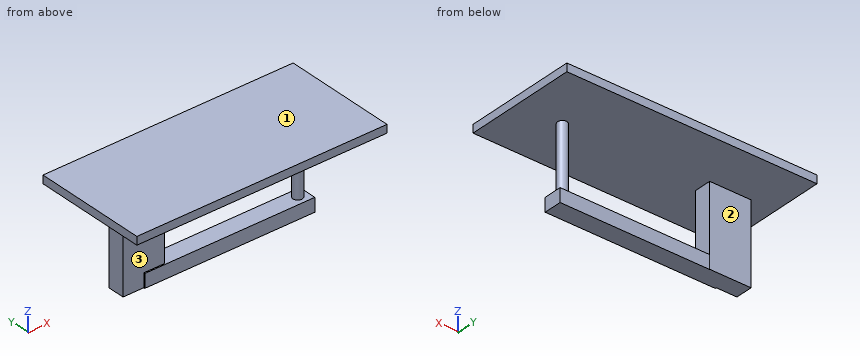
from build123d import *

# Parameters (mm, degrees)
F0_W     = 89.621424675
F0_H     = 36.9273871183
F1_DEPTH = 174.3299812078
F3_W     = 541.3100868464
F3_H     = 245.468556881
F4_DEPTH = 17.3550322652
F2_W     = 38.959980011
F2_H     = 29.5604169369
F5_DEPTH = 368.040561676
F6_R     = 10.2494359016
F7_DEPTH = 180.2812367678


with BuildPart() as f1:
    # F0 (on Top) → F1 (new body)
    with BuildSketch(Plane.XY):
        with Locations((0, 18.4636935592)):
            Rectangle(F0_W, F0_H)
    extrude(amount=F1_DEPTH)

    # F3 (on face) → F4 (join)
    with BuildSketch(Plane.XY.offset(174.3299812078)):
        with Locations((172.7937683463, 22.5193798542)):
            Rectangle(F3_W, F3_H)
    extrude(amount=F4_DEPTH)

    # F2 (on Right) → F5 (join)
    with BuildSketch(Plane.YZ):
        with Locations((16.8825984001, 14.7802084684)):
            Rectangle(F2_W, F2_H)
    extrude(amount=F5_DEPTH)

    # F6 (on face) → F7 (join)
    with BuildSketch(Plane(origin=(0, 0, 0), x_dir=(1, 0, 0), z_dir=(0, 0, -1))):
        with Locations((347.0340669155, -16.8822109699)):
            Circle(F6_R)
    extrude(amount=-F7_DEPTH)


solid = f1.part
The listing builds one solid part. Answer for the finished solid, in the listing's coordinates (mm). Face numbers are marked on the shaded views. Coordinates: 2 decimals unless noted, no trailing zeros. Write each loop counter-clockwise with the first axis right and the second up, starting at its lowest first coordinate (ties: lowest second). Pieces come first, ordered by that corner, then holes. Notation, with made-up numbers: (-32.75, 55) - (-22.75, 55) arc R13 cw to (-22.75, 72) - close; hole circle Ø9 at (52.5, 22). An arc over 180 degrees is marked (long way). Return JSON: item names as keys, results as strings.
1. The part is cut by section D-D on z = 141.5. Determine the outline of the cut face in (x, y).
Final values:
{"outline": "(-44.81, 0) - (44.81, 0) - (44.81, 36.93) - (-44.81, 36.93) - close; circle Ø20.5 at (347.03, 16.88)"}
2. The part is cut by section C-C on x = 32. Determine the outline of the cut face in (y, z).
Final values:
{"outline": "(-100.21, 174.33) - (0, 174.33) - (0, 29.56) - (-2.6, 29.56) - (-2.6, 0) - (36.93, 0) - (36.93, 174.33) - (145.25, 174.33) - (145.25, 191.69) - (-100.21, 191.69) - close"}
3. Consider line 1 along Z through (x, y) = (98.5, 9.5); line 2 along X through (y, z) = (30.5, 106.5); line 3 along Y through (x, z) = (-34.5, 144). Determine where each line is inside the solid, lowest interval first.
Final values:
{"line 1": "0 to 29.56, 174.33 to 191.69", "line 2": "-44.81 to 44.81", "line 3": "0 to 36.93"}
4. The part is cut by section B-B on z = 12.5. Determine the outline of the cut face in (x, y).
Final values:
{"outline": "(-44.81, 0) - (0, 0) - (0, -2.6) - (368.04, -2.6) - (368.04, 36.36) - (44.81, 36.36) - (44.81, 36.93) - (-44.81, 36.93) - close"}
5. For a pull along Z with two mould halves and no side action, classify the marked faces 1, 2 and 3 as +Z half, -Z half, draft (parallel to the pull), parting line (faces both ways), or undercut.
Final values:
{"face 1": "+Z half", "face 2": "draft", "face 3": "undercut"}
6. Each of these flat-tipped pins is pushed along its axis until it touches: pin 1 Ø23.5 at (x, z) = (248.5, 16) entering from +Y; pin 2 Ø0.8 at (y, z) = (-1.5, 21.5) entering from -X; pin 3 Ø5 at (x, y) = (55.5, 45.5) entering from -Z. Where does it stop, or does it pass through?
Final values:
{"pin 1": "y = 36.36", "pin 2": "x = 0", "pin 3": "z = 174.33"}
7. The part is cut by section A-A on x = 89. Determine the outline of the cut face in (y, z).
Final values:
{"outline": "(-100.21, 174.33) - (145.25, 174.33) - (145.25, 191.69) - (-100.21, 191.69) - close; (-2.6, 0) - (36.36, 0) - (36.36, 29.56) - (-2.6, 29.56) - close"}
